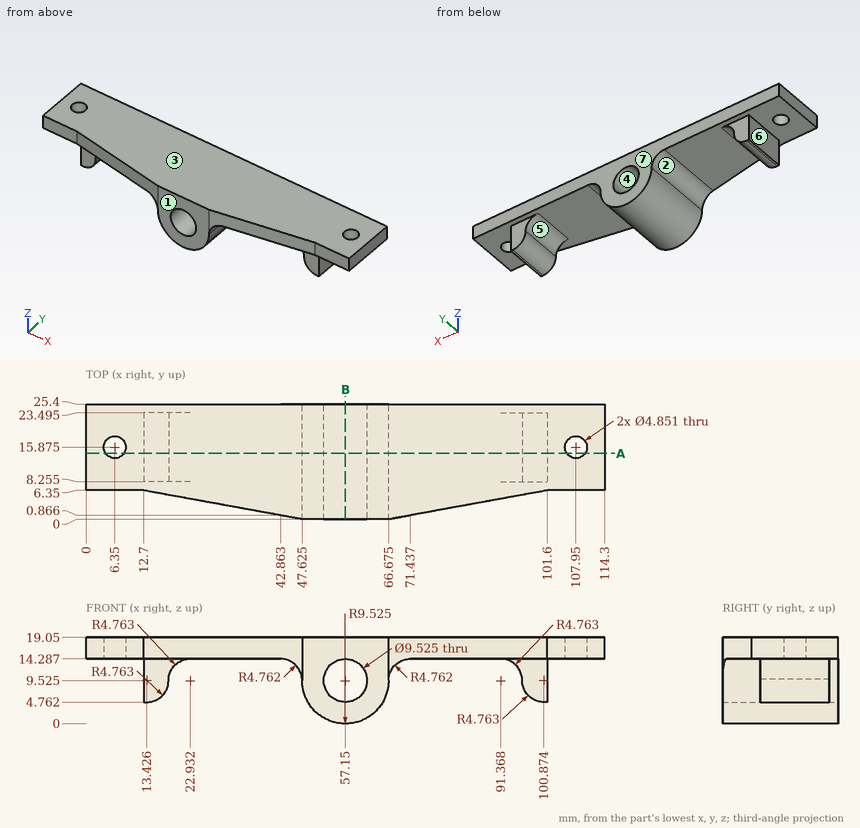
Job drawing, mm, ordinate dimensions from the low corner. One solid piece. A direction names the side the tool comes from. Round coordinates to 2 decimals unless told otherwise and drop trailing zeros. Write each loop counter-clockwise with the first axis right and the second up, starting at its lowest first coordinate (ties: lowest second). Pieces come first, ordered by that corner, then holes. Notation, with made-up numbers: M -32,-37.75 L -5,-37.75 A24 cw -5,-20.75 Z; hole C 62,34.5 d6. An arc over 180 degrees is marked long. Return JSON: item names as keys, results as strings. Group by question number.
(1) Saw through at A-A on y = 14.5. Count the separate pieces of the cut face and the enclosed holes in it.
(2) Pin check, flat tips, straight feed: pin 1 Ø5 at (x, z) = (17.5, 10.5) entering from +Y (1 decimal); pin 2 Ø6.5 at (x, y) = (107.95, 15.875) entering from +Z; pin 3 Ø1.5 at (x, y) = (77.5, 13.5) entering from -Z; pin 4 Ø7.5 at (x, z) = (20.5, 9) entering from -Y (1 decimal). Stop position of each tip, or through.
(3) Drill centre lines: probe 1 along Z at (x, y) = (57.15, 17); probe 2 along X at (y, z) = (16.25, 10); probe 3 along Y at (x, z) = (107.95, 17.65). Where is each one in solid material? Low to high.
(4) Saw through at B-B on x = 57.15. Write the cut outline in (y, z), then the cut area to 3 significant figures.
(5) Two-plate mould, pull along Z, no slides. Class the marked faces 1, 2, 3 and 4: +Z half, -Z half, draft (parallel to the pull), parting line (faces both ways), or undercut.
(6) Which spindle directions (+Z, -Z, +X, -X, +Y, -Y) get a long thin tool onto all of the face, cutting with end or side? Do the marked faces 5, 6 and 7. Say none if no direction does.
Returned:
{
 "1": {"separate pieces": "3", "enclosed holes": "1"},
 "2": {"pin 1": "y = 23.5", "pin 2": "z = 19.05", "pin 3": "z = 14.29", "pin 4": "y = 8.3"},
 "3": {"probe 1": "0 to 4.76, 14.29 to 19.05", "probe 2": "12.7 to 18.19, 47.6 to 52.41, 61.89 to 66.7, 96.11 to 101.6", "probe 3": "6.35 to 13.45, 18.3 to 25.4"},
 "4": {"outline": "M 0,0 L 25.4,0 L 25.4,4.76 L 0,4.76 Z; M 0,14.29 L 25.4,14.29 L 25.4,19.05 L 0,19.05 Z", "area": "242 mm²"},
 "5": {"face 1": "draft", "face 2": "-Z half", "face 3": "+Z half", "face 4": "undercut"},
 "6": {"face 5": "-Z, +Y, -Y", "face 6": "-Z, -X, +Y, -Y", "face 7": "+Z, -Z, +X, -X, +Y"}
}
